Build history of the part. All positions in model axes, mm. A direction names the side the tool comes from. Round coordinates to 2 decimals unless told otherwise and drop trailing zeros. Write each loop counter-clockwise with the first axis right and the second up, starting at its lowest first coordinate (ties: lowest second). Pieces come first, ordered by that corner, then holes.
Item 1: Band-saw the part on A-A, the plane x = 490. Write the cut outline in (y, z).
Item 2: Band-saw the part on B-B, the plane z = 290.5. Write the cut outline in (x, y), then the cut area to 3 significant figures.
Item 3: Wall check: probe 1 along Y at (x, z) = (612, 162.5); probe 2 along Z at (x, y) = (1022.5, -77.5). Give the ranges that are in metal, low to high.
Item 4: 3-axis set-ups, long thin cutter, end or side, ignore diameter. For faces 1 (the flat face through (601, -6.35, 255)), 2 (the flat face through (601, 0, 255)), 3 (the flat face through (597.553, -4, 91)): which of +Z, -Z, +X, -X, +Y, -Y reach the whole face in a straight line?
Item 5: Drop flat-ended pins along their axis: pin 1 Ø5 at (x, y) = (490.5, -4.5) entering from +Z; pin 2 Ø1.9 at (y, z) = (-3, 359.5) entering from +X; pin 3 Ø1.9 at (y, z) = (-4.5, 243) entering from +X. Give the stop position or say it passes through.
```python
from build123d import *

# Parameters (mm, degrees)
F1_DEPTH = 6.35
F2_DEPTH = 25
F4_DEPTH = 12.7


with BuildPart() as f1:
    # F0 (on Front) → F1 (new body)
    with BuildSketch(Plane.XZ):
        with BuildLine():
            Line((-31.097302, 79.375), (-31.097302, 0))
            Line((-31.097302, 0), (597.552698, 0))
            Line((597.552698, 0), (597.552698, 158.75))
            Line((597.552698, 158.75), (76.952726, 158.75))
            ThreePointArc((76.952726, 158.75), (10.848593, 135.505324), (-31.097302, 79.375))
        make_face()
        Polygon((597.552698, 158.75), (597.552698, 0), (617.552698, 0), (617.552698, 330.2), (617.552698, 347.6625), (597.552698, 347.6625), (597.552698, 330.2), align=None)
        Polygon((330.852698, 330.2), (597.552698, 330.2), (597.552698, 347.6625), (378.905624, 347.6625), (378.905624, 365.125), (360.092938, 365.125), align=None)
    extrude(amount=F1_DEPTH)

    # F0 (on Front) → F2 (cut)
    with BuildSketch(Plane.XZ):
        with BuildLine():
            Line((-31.097302, 79.375), (-31.097302, 0))
            Line((-31.097302, 0), (597.552698, 0))
            Line((597.552698, 0), (597.552698, 158.75))
            Line((597.552698, 158.75), (76.952726, 158.75))
            ThreePointArc((76.952726, 158.75), (10.848593, 135.505324), (-31.097302, 79.375))
        make_face()
    extrude(amount=F2_DEPTH, mode=Mode.SUBTRACT)

    # F3 (on face) → F4 (join)
    with BuildSketch(Plane(origin=(0, 0, 0), x_dir=(1, 0, 0), z_dir=(0, 0, -1))):
        Polygon((597.552698, 16.692741), (597.552698, 3.175), (597.552698, -225.425), (1054.752698, -225.425), (1054.752698, 231.775), (597.552698, 231.775), align=None)
    extrude(amount=-F4_DEPTH)


solid = f1.part
```
Results:
1. outline: (-6.35, 330.2) - (0, 330.2) - (0, 347.66) - (-6.35, 347.66) - close
2. outline: (597.55, -6.35) - (617.55, -6.35) - (617.55, 0) - (597.55, 0) - close
2. area: 127 mm2
3. probe 1: y = -6.35 to 0
3. probe 2: z = 0 to 12.7
4. face 1: +Z, +X, -X, -Y
4. face 2: +Z, +X, -X, +Y
4. face 3: -Z, -X, +Y, -Y
5. pin 1: stops at z = 347.66
5. pin 2: stops at x = 378.91
5. pin 3: stops at x = 617.55
